```python
from build123d import *

# Parameters (mm, degrees)
PAD001_DEPTH = 1


with BuildPart() as hinge:
    # Sketch003 → Pad001 (new body)
    with BuildSketch(Plane.XY):
        with BuildLine():
            Line((10, 0), (10, 1.9))
            ThreePointArc((10, 1.9), (9.787661, 2.445156), (9.261032, 2.7))
            Line((4.547651, 2.7), (9.261032, 2.7))
            Line((4.547651, 0), (4.547651, 2.7))
            Line((4.547651, 0), (4.547651, -2.7))
            Line((4.547651, -2.7), (9.228747, -2.7))
            ThreePointArc((9.228747, -2.7), (9.775939, -2.45576), (10, -1.9))
            Line((10, 0), (10, -1.9))
        make_face()
    extrude(amount=PAD001_DEPTH)


with BuildPart() as hinge_1:
    # Body003 placement: moved
    add(hinge.part.moved(Location((0, 0, 38))))


with BuildPart() as body_w_hinge:
    # Sketch001 → Revolution (revolve)
    with BuildSketch(Plane.XZ):
        with BuildLine():
            Line((0, 0), (0, 1.1))
            ThreePointArc((0, 1.1), (1.180458, 1.533416), (1.8, 2.627718))
            Line((1.8, 2.627718), (4.45, 18.712917))
            Line((4.45, 18.712917), (4.45, 38.9))
            Line((4.45, 38.9), (5.714157, 38.9))
            Line((5.714157, 38.9), (6.011811, 38.234338))
            ThreePointArc((5.716101, 37.9), (5.923028, 38.014921), (6.011811, 38.234338))
            Line((5.35, 37.9), (5.716101, 37.9))
            Line((5.35, 18.9), (5.35, 37.9))
            Line((2.599788, 2.206524), (5.35, 18.9))
            ThreePointArc((0, 0), (1.704967, 0.625994), (2.599788, 2.206524))
        make_face()
    revolve(axis=Axis((0, 0, 0), (0, 0, 1)))

    # Fusion: union Hinge
    add(hinge_1.part)


solid = body_w_hinge.part
```
Design review of the part built by this model. Coordinates are the model's own, in mm. A direction names the side the tool comes from. Give positions to 0.01 mm unless a question says otherwise; leave off trailing zeros. Order: outer loops, then holes, each group sorted by start corner. A loop starts at its lowest first (then second) coordinate and runs counter-clockwise, first axis right, second up. Notation, with made-up numbers: (2.5, 49.5) - (40.5, 49.5) arc R15 ccw to (40.5, 77.5) - close; hole circle Ø3 at (-35, 82.5). An arc over 180 degrees is marked (long way). Use a Markdown table: item, result. Add a question column.
(1) Machinability: for faces 5 (the face through (7, 0, 39)), 6 (the face through (-5.1, -2.1, 37.9)), which of the approach directions +Z, -Z, +X, -X, +Y, -Y give a long, thin tool a straight path to every point of the face, cutting with its end or side? Answer none if there is none.
(2) Add section C-C on z = 5. Give the boundary of the cut face in (x, y), then the cut area to 3 significant figures.
(3) Add section B-B on x = 8.25. Give the boundary of the cut face in (y, z), then the cut area to 3 significant figures.
(4) Add section A-A on z = 29. Give the boundary of the cut face in (x, y).
(5) Mouldability with a two-part tool opening along X and no side actions: class faces 1 (the face through (10, 0, 38.5)), 2 (the face through (-0.68, -3.07, 10.78)), 3 (the face through (7.4, 2.7, 38.5)), 4 (the face through (-0.965, -4.344, 28.948)) as +X half, -X half, draft (parallel to the pull), parting line (faces both ways), or undercut.
(6) Clearance check with flat-ended pins moving along their axes: P1, Ø4, axis at x = 3.5, y = 1.5, coming from the -Z side; P2, Ø1, axis at x = 4, y = 4.5, coming from the +Z side; P3, Ø2, axis at x = 2, z = 21, coming from the -Y side. State where each tip first meets the part, or that it passes through.
(7) Wall thickness on probe 1 along X at (y, z) = (0.25, 33); probe 2 along Y at (x, z) = (0, 28.25); probe 3 along Z at (x, y) = (5.5, 2.5): over which ranges is each line inside the solid? List them lowest first. Write a range as [from, to].
Report:
| question | item | result |
|---|---|---|
| 1 | face 5 | +Z, +X, -X, +Y, -Y |
| 1 | face 6 | -Z |
| 2 | outline | circle Ø6.12 at (0, 0); hole circle Ø4.38 at (0, 0) |
| 2 | area | 14.3 mm² |
| 3 | outline | (-2.7, 38) - (2.7, 38) - (2.7, 39) - (-2.7, 39) - close |
| 3 | area | 5.40 mm² |
| 4 | outline | circle Ø10.7 at (0, 0); hole circle Ø8.9 at (0, 0) |
| 5 | face 1 | +X half |
| 5 | face 2 | undercut |
| 5 | face 3 | draft |
| 5 | face 4 | undercut |
| 6 | P1 | stops at z = 0.72 |
| 6 | P2 | stops at z = 38.9 |
| 6 | P3 | stops at y = -5.26 |
| 7 | probe 1 | x = [-5.34, -4.44], [4.44, 5.34] |
| 7 | probe 2 | y = [-5.35, -4.45], [4.45, 5.35] |
| 7 | probe 3 | z = [38, 39] |
